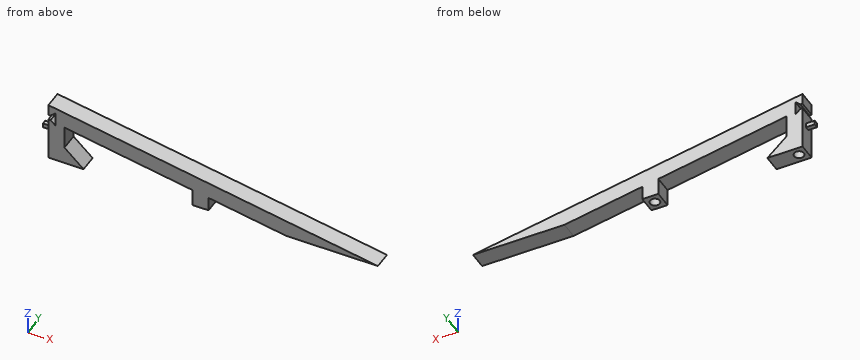
```python
from build123d import *

# Parameters (mm, degrees)
P_IDAT_VYSUNUT_M1_DEPTH  = 8
ODEBRAT_VYSUNUT_M1_DEPTH = 153.557332159
SKICA3_W                 = 2
SKICA3_H                 = 2
P_IDAT_VYSUNUT_M2_DEPTH  = 4
SKICA5_W                 = 16
SKICA5_H                 = 8
P_IDAT_VYSUNUT_M4_DEPTH  = 8
ODEBRAT_VYSUNUT_M3_DEPTH = 153.557332159
SKICA8_R                 = 2.2
ODEBRAT_VYSUNUT_M4_DEPTH = 9.4


with BuildPart() as part:
    # Skica1 → Přidat vysunutím1 (new body)
    with BuildSketch(Plane(origin=(0, 0, 0), x_dir=(1, 0, 0), z_dir=(0, 1, 0))):
        Polygon((0, 0), (0, -27.47211487), (149.85, 0.000769495), (108.259653873, 0.000769495), (72.85, -6.491091207), (72.85, 0), (65.55, 0), (65.55, -7.829443265), (7.3, -18.508759343), (7.3, 0), align=None)
    extrude(amount=P_IDAT_VYSUNUT_M1_DEPTH)

    # Skica2 → Odebrat vysunutím1 (cut, through all)
    with BuildSketch(Plane(origin=(0, 8, 0), x_dir=(1, 0, 0), z_dir=(0, 1, 0))):
        Polygon((0, -20), (1, -20), (3.2, -18), (3.2, -24.4), (1, -22.4), (0, -22.4), align=None)
    extrude(amount=-ODEBRAT_VYSUNUT_M1_DEPTH, mode=Mode.SUBTRACT)

    # Skica3 → Přidat vysunutím2 (add)
    with BuildSketch(Plane.ZY):
        with Locations((13.2, 4)):
            Rectangle(SKICA3_W, SKICA3_H)
    extrude(amount=P_IDAT_VYSUNUT_M2_DEPTH)

    # Skica5 → Přidat vysunutím4 (add)
    with BuildSketch(Plane(origin=(0, 8, 0), x_dir=(1, 0, 0), z_dir=(0, 1, 0))):
        with Locations((8, -4)):
            Rectangle(SKICA5_W, SKICA5_H)
    extrude(amount=-P_IDAT_VYSUNUT_M4_DEPTH)

    # Skica7 → Odebrat vysunutím3 (cut, through all)
    with BuildSketch(Plane.XZ):
        Polygon((7.3, 8), (16, 8), (16, 0), align=None)
    extrude(amount=-ODEBRAT_VYSUNUT_M3_DEPTH, mode=Mode.SUBTRACT)

    # Skica8 → Odebrat vysunutím4 (cut)
    with BuildSketch(Plane(origin=(0, 0, 0), x_dir=(-1, 0, 0), z_dir=(0, 0, -1))):
        with Locations((-3.65, 4)):
            Circle(SKICA8_R)
        with Locations((-69.2, 4)):
            Circle(SKICA8_R)
    extrude(amount=-ODEBRAT_VYSUNUT_M4_DEPTH, mode=Mode.SUBTRACT)


solid = part.part
```
Geometry: final body of the model. Coordinates: model frame, mm. Give positions to 0.01 mm unless a question says otherwise; leave off trailing zeros. Order: outer loops, then holes, each group sorted by start corner. A loop starts at its lowest first (then second) coordinate and runs counter-clockwise, first axis right, second up. Notation, with made-up numbers: (13, 8.25) -> (69, 8.25) arc R23 cw to (69, 45.25) -> close; hole circle Ø5 at (55, -25.75). An arc over 180 degrees is marked (long way). Write each question's results on one line, items separated by ' | '. Start each with the question number.
1) Section B-B (x = 69.2). Return loops of the section in (y, z), then the cut area to 3 significant figures.
2) Line query: line 1 (Y direction, x = 69.2, z = 7.75); line 2 (Z direction, x = 122.5, y = 7); line 3 (Z direction, x = 64.5, y = 2). Output: solid intervals per line, ascending. Write a range as from..to.
3) First-contact query: pin 1 (4 mm diameter, centred on y = 5, z = 26, fed in from -X); pin 2 (0.6 mm diameter, centred on x = -2, y = 3.5, fed in from -Z); pin 3 (3 mm diameter, centred on x = 103, y = 4, fed in from +Z). Flat tips, straight axial feed; report the tip coordinate or a pass-through.
4) Section C-C (x = 131.5). Return loops of the section in (y, z).
5) Section A-A (z = 2). Return loops of the section in (x, y) (3 decimals), then the cut area to 3 significant figures.
Calculated:
1) outline: (0, 0) -> (1.8, 0) -> (1.8, 9.4) -> (6.2, 9.4) -> (6.2, 0) -> (8, 0) -> (8, 14.79) -> (0, 14.79) -> close | area: 76.9 mm2
2) line 1: 0..1.8, 6.2..8 | line 2: 0..5.01 | line 3: 8.02..15.65
3) pin 1: x = 0 | pin 2: z = 12.2 | pin 3: z = 8.86
4) outline: (0, 0) -> (8, 0) -> (8, 3.36) -> (0, 3.36) -> close
5) outline: (0, 0) -> (13.825, 0) -> (13.825, 8) -> (0, 8) -> close; (65.55, 0) -> (72.85, 0) -> (72.85, 8) -> (65.55, 8) -> close; (97.347, 0) -> (138.937, 0) -> (138.937, 8) -> (97.347, 8) -> close; hole circle Ø4.4 at (3.65, 4); hole circle Ø4.4 at (69.2, 4) | area: 471 mm2
